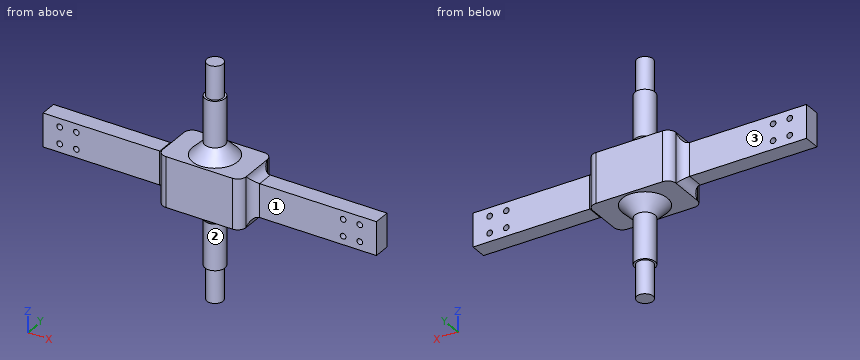
```python
from build123d import *

# Parameters (mm, degrees)
SKETCH1_W            = 200
SKETCH1_H            = 20
BOSS_EXTRUDE1_DEPTH  = 5
SKETCH2_W            = 50
SKETCH2_H            = 30
BOSS_EXTRUDE2_DEPTH  = 15
FILLET3_R            = 5
SKETCH3_R            = 6
BOSS_EXTRUDE3_DEPTH  = 50
CHAMFER1_SIZE        = 7.5
M3_CLEARANCE_HOLE1_D = 3.4
SKETCH19_R           = 4.825
BOSS_EXTRUDE4_DEPTH  = 20
BOSS_EXTRUDE5_START  = 20
SKETCH20_R           = 4.825
BOSS_EXTRUDE5_DEPTH  = 20


with BuildPart() as part:
    # Sketch1 → Boss-Extrude1 (new, symmetric)
    with BuildSketch(Plane(origin=(0, 0, 0), x_dir=(1, 0, 0), z_dir=(0, 1, 0))):
        Rectangle(SKETCH1_W, SKETCH1_H)
    extrude(amount=BOSS_EXTRUDE1_DEPTH, both=True)

    # Sketch2 → Boss-Extrude2 (add, symmetric)
    with BuildSketch(Plane.XY):
        Rectangle(SKETCH2_W, SKETCH2_H)
    extrude(amount=BOSS_EXTRUDE2_DEPTH, both=True)

    # Fillet3
    fillet3_edges = [part.edges().sort_by_distance(p)[0] for p in [
        (-25, -5, 0),
        (25, -5, 0),
        (25, -15, 0),
        (25, 0, 10),
        (25, 5, 0),
        (25, 0, -10),
        (-25, 15, 0),
        (-25, 0, -10),
        (-25, 5, 0),
        (-25, 0, 10),
        (25, 15, 0),
        (-25, -15, 0),
    ]]
    fillet(fillet3_edges, radius=FILLET3_R - 0.0001)  # a hair under: the kernel refuses the full size

    # Sketch3 → Boss-Extrude3 (add, symmetric)
    with BuildSketch(Plane.XY):
        with Locations(Location((0, 0, 0), (0, 0, 180))):
            Circle(SKETCH3_R)
    extrude(amount=BOSS_EXTRUDE3_DEPTH, both=True)

    # Chamfer1
    chamfer1_edges = [part.edges().sort_by_distance(p)[0] for p in [
        (6, 0, 15),
        (6, 0, -15),
    ]]
    chamfer(chamfer1_edges, length=CHAMFER1_SIZE)

    # M3 Clearance Hole1 (through all)
    with Locations(Plane(origin=(0, 5, 0), x_dir=(1, 0, 0), z_dir=(0, 1, 0))):
        with Locations((-90, 5), (-90, -5), (90, -5), (90, 5), (-80, 5), (-80, -5), (80, 5), (80, -5)):
            Hole(M3_CLEARANCE_HOLE1_D / 2)

    # Sketch19 → Boss-Extrude4 (add)
    with BuildSketch(Plane(origin=(0, 0, -50), x_dir=(-1, 0, 0), z_dir=(0, 0, -1))):
        Circle(SKETCH19_R)
    extrude(amount=BOSS_EXTRUDE4_DEPTH)

    # Sketch20 → Boss-Extrude5 (add)
    with BuildSketch(Plane.XY.offset(50).offset(BOSS_EXTRUDE5_START)):
        with Locations(Location((0, 0, 0), (0, 0, 180))):
            Circle(SKETCH20_R)
    extrude(amount=-BOSS_EXTRUDE5_DEPTH)


solid = part.part
```
Here's how the part is built. I have some questions about the finished solid (model axes, mm). Face numbers are marked on the shaded views. A direction names the side the tool comes from. Round coordinates to 2 decimals unless told otherwise and drop trailing zeros. Order: outer loops, then holes, each group sorted by start corner. A loop starts at its lowest first (then second) coordinate and runs counter-clockwise, first axis right, second up. Notation, with made-up numbers: M -12,65.25 L -6,65.25 A23 ccw -6,76.25 Z; hole C -6.75,27 d6. An arc over 180 degrees is marked long. Answer as CSV lines item,"result".
Item 1: Which directions (+Z, -Z, +X, -X, +Y, -Y) give clear straight access to the entire face, cutting with the end or side of a thin tool? Please do the marked faces 1, 2 and 3.
From the geometry:
face 1,"+Z, -Z, +X, -Y"
face 2,"-Z"
face 3,"+Z, -Z, -X, +Y"
Item 2: Imagine slicing it at C-C on x = 71.5. List the corners of the cut face in (y, z) for me.
From the geometry:
outline,"M -5,-10 L 5,-10 L 5,10 L -5,10 Z"
Item 3: Imagine slicing it at A-A on y = 0. Give the number of separate pieces and of enclosed holes in the cut face, and give its area (3 significant figures).
From the geometry:
separate pieces,"1"
enclosed holes,"8"
area,"5,790 mm2"
Item 4: Imagine slicing it at B-B on z = -18. List the corners of the cut face in (x, y) for me.
From the geometry:
outline,"C 0,0 d21"
Item 5: For pin 1 (3 mm diameter, centred on x = 50, y = -0.5, fed in from -Z); pin 2 (1.5 mm diameter, centred on y = -5, z = -51.5, fed in from +X); pin 3 (10 mm diameter, centred on x = 75.5, z = 2.5, fed in from -Y), each with a flat end and sliding along its axis, tell me the tip position at first contact or that it passes through.
From the geometry:
pin 1,"z = -10"
pin 2,"x = 2.28"
pin 3,"y = -5"
Item 6: Please list where these lines run through material, in increasing order: L1, parallel to X at y = -0.5, z = 5; L2, parallel to Z at x = 80, y = -1; L3, parallel to Z at x = -15, y = -1.25. Write a range as [from, to].
From the geometry:
L1,"[-100, -91.7], [-88.3, -81.7], [-78.3, 78.3], [81.7, 88.3], [91.7, 100]"
L2,"[-10, -6.7], [-3.3, 3.3], [6.7, 10]"
L3,"[-15, 15]"
Item 7: Imagine slicing it at D-D on z = -46.5. List the corners of the cut face in (x, y) for me.
From the geometry:
outline,"C 0,0 d12"
